Geometry check sheet. Reference: drawing and pictorial views, mm from the part's lowest x, y, z. A direction names the side the tool comes from. Give positions to 0.01 mm unless a question says otherwise; leave off trailing zeros. Order: outer loops, then holes, each group sorted by start corner. A loop starts at its lowest first (then second) coordinate and runs counter-clockwise, first axis right, second up.
Item 1: Material ranges on line 1 along Y through (x, z) = (36, 5); line 2 along Z through (x, y) = (28, 19.5) (1 decimal); line 3 along Z through (x, y) = (35, 12) (1 decimal), recorded low to high.
Item 2: Release check for a two-part mould opening along Z. For the marked faces 6, 7 and 8 record: released by +Z, released by -Z, zero draft, split by the parting line, or undercut.
Item 3: Sectioned sample at C-C on y = 11. Record the boundary of the cut face in (x, z) (1 decimal), and give its area (3 significant figures).
Item 4: Sectioned sample at B-B on x = 38.5. Record the boundary of the cut face in (y, z) (1 decimal).
Item 5: Sectioned sample at A-A on z = 5. Record the boundary of the cut face in (x, y).
Item 6: Access from +Z, -Z, +X, -X, +Y, -Y to the whole of each face (thin tool, end or side, straight path). Record for the marked faces 1, 2, 3, 4 and 5.
Item 7: Sectioned sample at D-D on x = 5. Record the boundary of the cut face in (y, z), and give its area (3 significant figures).
Item 8: Gauge pin test, flat ends, axial feed: P1, Ø1, axis at x = 22, z = 23, coming from the +Y side; P2, Ø7, axis at x = 12.5, z = 28.5, coming from the +Y side; P3, Ø10, axis at y = 20, z = 10.5, coming from the -X side (1 decimal). Record the tip position at first contact, or that the pin passes through.
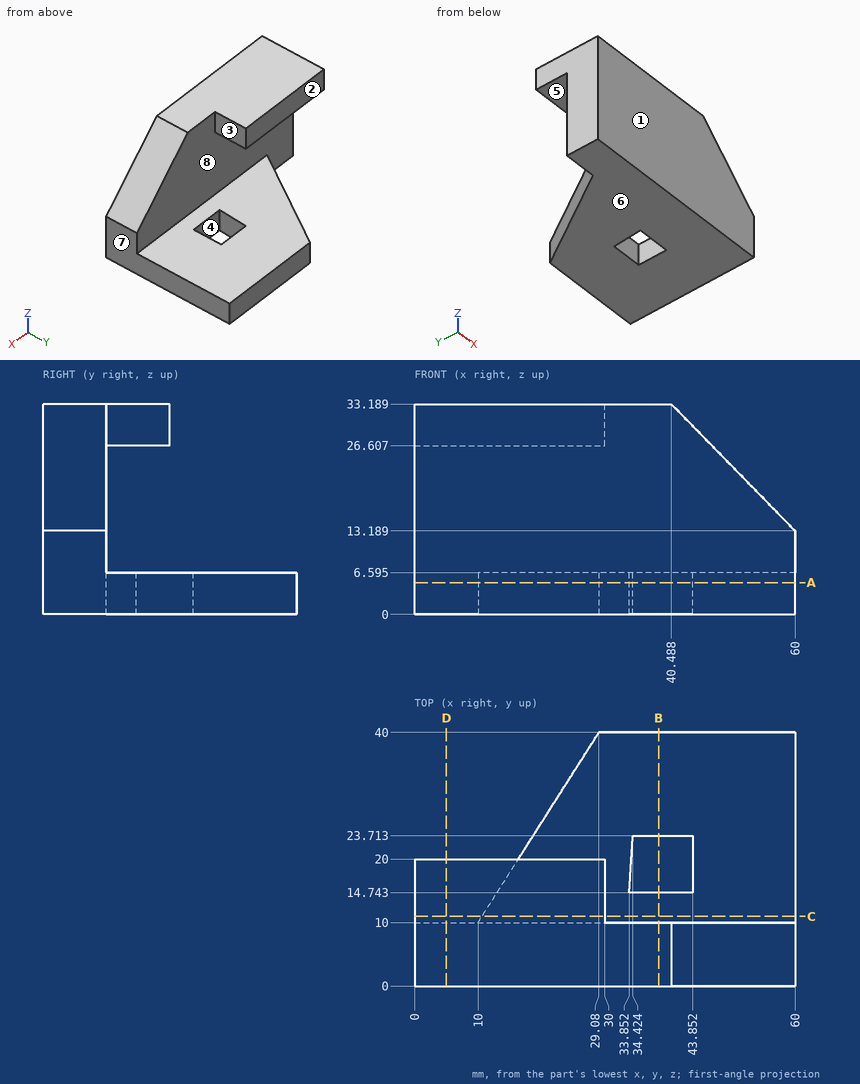
Report:
1. line 1: y = 0 to 14.74, 23.71 to 40
1. line 2: z = 0 to 6.6, 26.6 to 33.2
1. line 3: z = 0 to 6.6
2. face 6: released by -Z
2. face 7: zero draft
2. face 8: undercut
3. outline: (0, 26.6) - (30, 26.6) - (30, 33.2) - (0, 33.2) - close; (10.6, 0) - (60, 0) - (60, 6.6) - (10.6, 6.6) - close
3. area: 523 mm2
4. outline: (0, 0) - (14.7, 0) - (14.7, 6.6) - (10, 6.6) - (10, 33.2) - (0, 33.2) - close; (23.7, 0) - (40, 0) - (40, 6.6) - (23.7, 6.6) - close
5. outline: (0, 0) - (60, 0) - (60, 40) - (29.08, 40) - (10, 10) - (0, 10) - close; hole (33.85, 14.74) - (43.85, 14.74) - (43.85, 23.71) - (34.42, 23.71) - close
6. face 1: +Z, -Z, +X, -X, -Y
6. face 2: +Z, +X, -X, +Y
6. face 3: +Z, +X, +Y
6. face 4: +Z, -Z
6. face 5: +X, -X, +Y
7. outline: (0, 0) - (10, 0) - (10, 26.61) - (20, 26.61) - (20, 33.19) - (0, 33.19) - close
7. area: 398 mm2
8. P1: stops at y = 10
8. P2: stops at y = 20
8. P3: stops at x = 14.4
